from build123d import *

# Parameters (mm, degrees)
IZIM1_R                     = 2.85
IZIM1_R_2                   = 1.65
Y_KSEKLIK_EKSTR_ZYON1_DEPTH = 40
PAH1_SIZE                   = 0.2


with BuildPart() as part:
    # Çizim1 → Yükseklik-Ekstrüzyon1 (new body)
    with BuildSketch(Plane(origin=(0, 0, 0), x_dir=(1, 0, 0), z_dir=(0, 1, 0))):
        with Locations(Location((0, 0, 0), (0, 0, 270))):
            Circle(IZIM1_R)
        with Locations(Location((0, 0, 0), (0, 0, 270))):
            Circle(IZIM1_R_2, mode=Mode.SUBTRACT)
    extrude(amount=Y_KSEKLIK_EKSTR_ZYON1_DEPTH)

    # Pah1
    pah1_edges = [part.edges().sort_by_distance(p)[0] for p in [
        (0, 0, -2.85),
        (0, 40, -2.85),
        (0, 0, -1.65),
        (0, 40, -1.65),
    ]]
    chamfer(pah1_edges, length=PAH1_SIZE)


solid = part.part
Part model, mm, in its own coordinate system. Coordinates: 2 decimals unless noted, no trailing zeros. Loops run counter-clockwise (first coordinate to the right, second up) from the corner with the lowest first, then second, coordinate; pieces in that order, holes last. Notation, with made-up numbers: M 57,48.5 L 99,48.5 A17 ccw 99,74.5 Z; hole C -31,41 d3. An arc over 180 degrees is marked long. Use a Markdown table: item, result. Add a question column.
Q1. Pin check, flat tip, straight feed: P1, Ø1.5, axis at y = 33, z = -2, coming from the -X side. Stop position of the tip, or through.
Q2. Probe L1, parallel to X at y = 15, z = 0; L2, parallel to Z at x = 1.2, y = 32. List the from-to ranges inside material, lowest first.
Q3. Cut at C-C (y = 24). Write the cut outline in (x, z), and give its area (3 significant figures).
Q4. Cut at A-A (z = 0). Write the cut outline in (x, y).
Q5. Cut at B-B (x = 0). Write the cut outline in (y, z).
Q6. Mould opens along X. For faces 1 (the cylindrical face through (-1, 19.72, -1.31)), 2 (the cylindrical face through (-1.734, 19.723, -2.262)), 3 (the flat face through (2, 0, 1)) say: +X half, -X half, draft (parallel to the pull), parting line (faces both ways), or undercut.
Worked out:
| question | item | result |
|---|---|---|
| 1 | P1 | stops at x = -2.56 |
| 2 | L1 | x = -2.85 to -1.65, 1.65 to 2.85 |
| 2 | L2 | z = -2.59 to -1.13, 1.13 to 2.59 |
| 3 | outline | C 0,0 d5.7; hole C 0,0 d3.3 |
| 3 | area | 17.0 mm2 |
| 4 | outline | M -2.85,0.2 L -2.65,0 L -1.85,0 L -1.65,0.2 L -1.65,39.8 L -1.85,40 L -2.65,40 L -2.85,39.8 Z; M 1.65,0.2 L 1.85,0 L 2.65,0 L 2.85,0.2 L 2.85,39.8 L 2.65,40 L 1.85,40 L 1.65,39.8 Z |
| 5 | outline | M 0,-2.65 L 0.2,-2.85 L 39.8,-2.85 L 40,-2.65 L 40,-1.85 L 39.8,-1.65 L 0.2,-1.65 L 0,-1.85 Z; M 0,1.85 L 0.2,1.65 L 39.8,1.65 L 40,1.85 L 40,2.65 L 39.8,2.85 L 0.2,2.85 L 0,2.65 Z |
| 6 | face 1 | undercut |
| 6 | face 2 | parting line |
| 6 | face 3 | draft |
